```python
from build123d import *

# Parameters (mm, degrees)
SKETCH1_W               = 23.876
SKETCH1_H               = 35.052
SKETCH1_R               = 1.143
SKETCH1_R_2             = 0.635
BOSS_EXTRUDE1_DEPTH     = 3.175
SKETCH2_W               = 6.35
SKETCH2_H               = 9.652
BOSS_EXTRUDE2_DEPTH     = 9.525
SKETCH3_R               = 1.143
CUT_EXTRUDE2_DEPTH      = 36.052
CUT_EXTRUDE2_DEPTH_BACK = 6.35


with BuildPart() as part:
    # Sketch1 → Boss-Extrude1 (new body)
    with BuildSketch(Plane.XY):
        with Locations((11.938, 17.526)):
            Rectangle(SKETCH1_W, SKETCH1_H)
        with Locations((6.858, 11.938)):
            Circle(SKETCH1_R, mode=Mode.SUBTRACT)
        with Locations((17.018, 11.938)):
            Circle(SKETCH1_R, mode=Mode.SUBTRACT)
        with Locations((20.066, 17.526)):
            Circle(SKETCH1_R_2, mode=Mode.SUBTRACT)
        with Locations((3.81, 17.526)):
            Circle(SKETCH1_R_2, mode=Mode.SUBTRACT)
    extrude(amount=BOSS_EXTRUDE1_DEPTH)

    # Sketch2 → Boss-Extrude2 (add)
    with BuildSketch(Plane.XY):
        with Locations((11.938, 17.526)):
            Rectangle(SKETCH2_W, SKETCH2_H)
    extrude(amount=BOSS_EXTRUDE2_DEPTH)

    # Sketch3 → Cut-Extrude2 (cut, two sides)
    with BuildSketch(Plane(origin=(0, 0, 0), x_dir=(1, 0, 0), z_dir=(0, 1, 0))) as cut_extrude2_sk:
        with Locations((11.938, -6.35)):
            Circle(SKETCH3_R)
        with BuildLine():
            ThreePointArc((11.938, -9.525), (9.69293597, -8.59506403), (8.763, -6.35))
            Line((8.763, -6.35), (8.763, -9.525))
            Line((8.763, -9.525), (11.938, -9.525))
        make_face()
        with BuildLine():
            ThreePointArc((15.113, -6.35), (14.18306403, -8.59506403), (11.938, -9.525))
            Line((11.938, -9.525), (15.113, -9.525))
            Line((15.113, -9.525), (15.113, -6.35))
        make_face()
    extrude(amount=CUT_EXTRUDE2_DEPTH, mode=Mode.SUBTRACT)
    extrude(cut_extrude2_sk.sketch, amount=-CUT_EXTRUDE2_DEPTH_BACK, mode=Mode.SUBTRACT)


solid = part.part
```
Model file for the job. Use its own axes, mm. A direction names the side the tool comes from. Give positions to 0.01 mm unless a question says otherwise; leave off trailing zeros. Loops run counter-clockwise (first coordinate to the right, second up) from the corner with the lowest first, then second, coordinate; pieces in that order, holes last. Notation, with made-up numbers: (86, 81.25) - (129, 81.25) arc R21 cw to (129, 86.25) - close; hole circle Ø10 at (8.25, 48.25). An arc over 180 degrees is marked (long way). One line per item, written item: value. Start each with the question number.
1. Slice it at D-D (x = 9.75). List the corners of the cut face in (y, z) (3 decimals).
2. Pin check, flat tips, straight feed: pin 1 (3.5 mm diameter, centred on x = 11.938, z = 6.35, fed in from -Y); pin 2 (3 mm diameter, centred on x = 21, z = 3.5, fed in from -Y); pin 3 (2.5 mm diameter, centred on x = 17.018, y = 11.938, fed in from +Z) (3 decimals); pin 4 (1.4 mm diameter, centred on x = 6.858, y = 11.938, fed in from +Z). Stop position of each tip, or through.
3. Which spindle directions (+Z, -Z, +X, -X, +Y, -Y) get a long thin tool onto all of the face, cutting with end or side? Do faces 1 (the cylindrical face through (3.727, 18.156, 1.565)), 2 (the flat face through (12, 22.352, 5)), 3 (the flat face through (12, 12.7, 5)). Say none if no direction does.
4. Slice it at C-C (x = 6.75). List the corners of the cut face in (y, z) (3 decimals), plus the area to 3 significant figures.
5. Pull direction X, two halves, no side cores. Call faces 4 (the flat face through (12, 35.052, 2)), 5 (the flat face through (15.113, 17, 5)), 6 (the flat face through (8.763, 17, 5)), 7 (the cylindrical face through (12.994, 17.458, 6.788)): pulls with the +X half, pulls with the -X half, needs draft (parallel to the pull), parting line crosses it, or undercut.
6. Slice it at B-B (y = 16). List the corners of the cut face in (x, z) (3 decimals), plus the area to 3 significant figures.
7. Probe L1, parallel to X at y = 17, z = 2.25; L2, parallel to Z at x = 4, y = 11 (3 decimals); L3, parallel to X at y = 11.5, z = 1.75. List the from-to ranges inside material, lowest first. Write a range as from..to.
8. Slice it at A-A (x = 3.81). List the corners of the cut face in (y, z) (3 decimals).
Solution:
1. outline: (0, 0) - (35.052, 0) - (35.052, 3.175) - (22.352, 3.175) - (22.352, 8.651) - (12.7, 8.651) - (12.7, 3.175) - (0, 3.175) - close
2. pin 1: stops at y = 12.7
2. pin 2: stops at y = 0
2. pin 3: stops at z = 3.175
2. pin 4: passes through
3. face 1: +Z, -Z
3. face 2: +Z, +X, -X, +Y
3. face 3: +Z, +X, -X, -Y
4. outline: (0, 0) - (10.8, 0) - (10.8, 3.175) - (0, 3.175) - close; (13.076, 0) - (35.052, 0) - (35.052, 3.175) - (13.076, 3.175) - close
4. area: 104 mm^2
5. face 4: needs draft
5. face 5: pulls with the +X half
5. face 6: pulls with the -X half
5. face 7: undercut
6. outline: (0, 0) - (23.876, 0) - (23.876, 3.175) - (15.113, 3.175) - (15.113, 6.35) arc R3.175 ccw to (8.763, 6.35) - (8.763, 3.175) - (0, 3.175) - close; hole circle Ø2.286 at (11.938, 6.35)
6. area: 108 mm^2
7. L1: x = 0..3.45, 4.17..19.71, 20.42..23.88
7. L2: z = 0..3.175
7. L3: x = 0..5.8, 7.91..15.96, 18.07..23.88
8. outline: (0, 0) - (16.891, 0) - (16.891, 3.175) - (0, 3.175) - close; (18.161, 0) - (35.052, 0) - (35.052, 3.175) - (18.161, 3.175) - close
